Design review of the part built by this model. Coordinates are the model's own, in mm. Face numbers are marked on the shaded views. A direction names the side the tool comes from. Coordinates: 2 decimals unless noted, no trailing zeros. Loops run counter-clockwise (first coordinate to the right, second up) from the corner with the lowest first, then second, coordinate; pieces in that order, holes last. Notation, with made-up numbers: (46, 60.25) -> (74, 60.25) arc R19 cw to (74, 75.25) -> close; hole circle Ø9 at (-8, -7.5). An arc over 180 degrees is marked (long way). Use a Markdown table: item, result. Add a question column.
Q1. Take a section at B-B on y = 10.75. Write out the cut boundary in (x, z).
Q2. For the marked faces 5 and 6, list the 3-axis set-ups (+Z, -Z, +X, -X, +Y, -Y) from which the entire face can be reached by the end or side of a thin tool; tool diameter is ignored.
Q3. Clearance check with a flat-ended pin moving along its axis: pin 1 Ø1.2 at (x, z) = (-2.5, -0.5) entering from +Y. State where the tip first meets the part, or that it passes through.
Q4. Draft analysis for pull direction Z (two halves, no side actions). For the marked faces 1, 2, 3 and 4, state which applies: pulls with the +Z half, pulls with the -Z half, needs draft (parallel to the pull), parting line crosses it, or undercut.
Q5. For probe 1 along X at (y, z) = (7.5, -1.9); probe 2 along Z at (x, y) = (-1.25, 10); probe 3 along Z at (x, y) = (-3.75, -1), list the stretches that pass through material, from the lowest coordinate up.
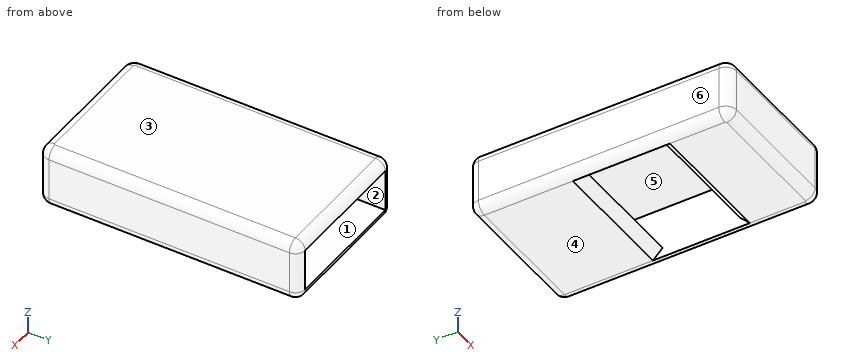
from build123d import *

# Parameters (mm, degrees)
F1_DEPTH    = 2.85
F2_DEPTH    = 1.95
F3_DEPTH    = 2.85
F4_DEPTH    = 1.95
F5_R        = 1
F7_DEPTH    = 25
F8_T1_DEPTH = 11.9
F9_R        = 0.89999


# Not quite as in the source:
# - a fillet or chamfer that OpenCascade refuses, or shapes differently, is made with other operations: its cross-section is extruded or revolved along the edge and cut away or added
# - a fillet or chamfer is up to 0.001 mm smaller than in the source, because OpenCascade refuses the exact size


with BuildPart() as f1:
    # F0 (on Top) → F1 (new body)
    with BuildSketch(Plane.XY):
        Polygon((-5.95, 11.2), (-5.95, -11.2), (5.95, -11.2), (5.95, 11.2), (5.95, 12.1), (-5.95, 12.1), align=None)
        Polygon((5.95, -11.2), (-5.95, -11.2), (-5.95, 11.2), (-5.95, 12.1), (-6.85, 12.1), (-6.85, -12.1), (6.85, -12.1), (6.85, 12.1), (5.95, 12.1), (5.95, 11.2), align=None)
    extrude(amount=F1_DEPTH)

    # F0 (on Top) → F2 (cut)
    with BuildSketch(Plane.XY):
        Polygon((-5.95, 11.2), (-5.95, -11.2), (5.95, -11.2), (5.95, 11.2), (5.95, 12.1), (-5.95, 12.1), align=None)
    extrude(amount=F2_DEPTH, mode=Mode.SUBTRACT)

    # F0 (on Top) → F3 (join)
    with BuildSketch(Plane.XY):
        Polygon((-5.95, 11.2), (-5.95, -11.2), (5.95, -11.2), (5.95, 11.2), (5.95, 12.1), (-5.95, 12.1), align=None)
        Polygon((5.95, -11.2), (-5.95, -11.2), (-5.95, 11.2), (-5.95, 12.1), (-6.85, 12.1), (-6.85, -12.1), (6.85, -12.1), (6.85, 12.1), (5.95, 12.1), (5.95, 11.2), align=None)
    extrude(amount=-F3_DEPTH)

    # F0 (on Top) → F4 (cut)
    with BuildSketch(Plane.XY):
        Polygon((-5.95, 11.2), (-5.95, -11.2), (5.95, -11.2), (5.95, 11.2), (5.95, 12.1), (-5.95, 12.1), align=None)
    extrude(amount=-F4_DEPTH, mode=Mode.SUBTRACT)

    # F5
    f5_edges = [f1.edges().sort_by_distance(p)[0] for p in [
        (5.95, -11.2, 0),
        (-5.95, -11.2, 0),
        (-6.85, -12.1, 0),
        (6.85, -12.1, 0),
    ]]
    fillet(f5_edges, radius=F5_R)

    # F6 (on Top) → F7 (cut)
    with BuildSketch(Plane.XY):
        Polygon((-5.95, 1), (-5.95, -4), (5.95, -4), (5.95, 1), (0, 1), align=None)
    extrude(amount=-F7_DEPTH, mode=Mode.SUBTRACT)

    # F8: chamfer of 2 on 2 edges, made by hand

    # F8_s2 → F8_t1 (cut)
    with BuildSketch(Plane.YZ.offset(-5.95)):
        Polygon((-6, -2.85), (-4, -0.85), (-4, -2.85), align=None)
        Polygon((3, -2.85), (1, -0.85), (1, -2.85), align=None)
    extrude(amount=F8_T1_DEPTH, mode=Mode.SUBTRACT)

    # F9 (radius 0.9 in the source; OpenCascade refuses exactly that, so slightly less here)
    f9_edges = [f1.edges().sort_by_distance(p)[0] for p in [
        (6.85, 12.1, 0),
        (-6.85, 12.1, 0),
        (0, 12.1, -2.85),
        (0, 12.1, 2.85),
        (6.85, 0.5, -2.85),
        (0, -12.1, 2.85),
        (-6.85, 0.5, 2.85),
        (-6.85, 0.5, -2.85),
        (-6.557107, -11.807107, -2.85),
        (0, -12.1, -2.85),
        (6.557107, -11.807107, -2.85),
        (6.85, 0.5, 2.85),
        (6.557107, -11.807107, 2.85),
        (-6.557107, -11.807107, 2.85),
    ]]
    fillet(f9_edges, radius=F9_R)


solid = f1.part
Answer list:
| question | item | result |
|---|---|---|
| 1 | outline | (-6.85, -1.95) arc R0.9 ccw to (-5.95, -2.85) -> (5.95, -2.85) arc R0.9 ccw to (6.85, -1.95) -> (6.85, 1.95) arc R0.9 ccw to (5.95, 2.85) -> (-5.95, 2.85) arc R0.9 ccw to (-6.85, 1.95) -> close; hole (-5.95, -1.95) -> (5.95, -1.95) -> (5.95, 1.95) -> (-5.95, 1.95) -> close |
| 2 | face 5 | +Y |
| 2 | face 6 | +Z, -Z, -X, +Y, -Y |
| 3 | pin 1 | y = -11.2 |
| 4 | face 1 | undercut |
| 4 | face 2 | undercut |
| 4 | face 3 | pulls with the +Z half |
| 4 | face 4 | pulls with the -Z half |
| 5 | probe 1 | -6.85 to -5.95, 5.95 to 6.85 |
| 5 | probe 2 | -2.85 to -1.95, 1.95 to 2.85 |
| 5 | probe 3 | 1.95 to 2.85 |
